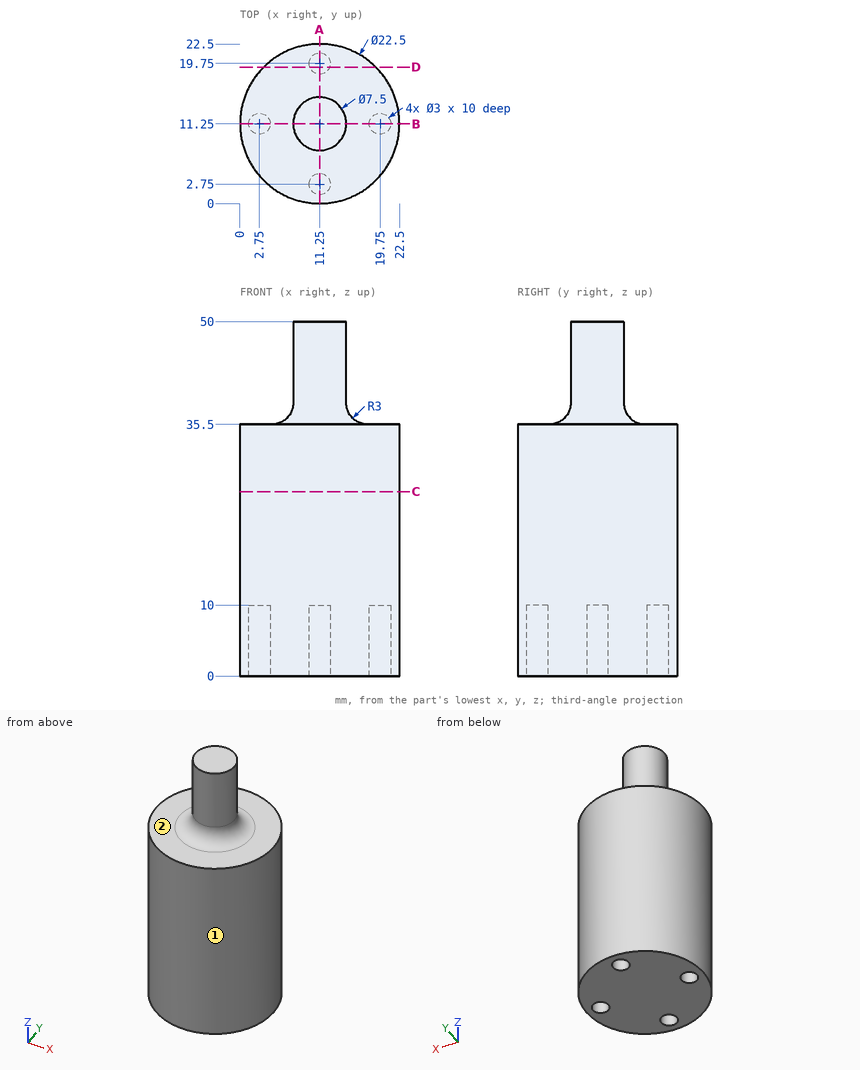
For this review, use the dimensioned drawing (mm, ordinates from the lowest corner) and the shaded views. A direction names the side the tool comes from. Round coordinates to 2 decimals unless told otherwise and drop trailing zeros. Order: outer loops, then holes, each group sorted by start corner. A loop starts at its lowest first (then second) coordinate and runs counter-clockwise, first axis right, second up. Notation, with made-up numbers: M 18.5,77 L 33.5,77 A26 cw 33.5,114 Z; hole C 40,42 d9. An arc over 180 degrees is marked long. Use a Markdown table: item, result. Add a question column.
Item 1: To check wall thickness, follow line 1 along Y through (x, z) = (11.25, 3); line 2 along Z through (x, y) = (10.25, 4.75); line 3 along Y through (x, z) = (19.75, 2.5). State the ranges of each line that lie inside material, in increasing order.
Item 2: Tool access review of the marked faces 1 and 2: name each direction out of +Z, -Z, +X, -X, +Y, -Y from which nothing blocks a thin tool from reaching the whole face with its end or side.
Item 3: Add section D-D, the plane y = 19.25. Give the boundary of the cut face in (x, z), then the cut area to 3 significant figures.
Item 4: Add section A-A, the plane x = 11.25. Give the boundary of the cut face in (y, z).
Item 5: Insertion check: pin 1 (6 mm diameter, centred on x = 2.5, y = 19, fed in from +Z); pin 2 (1.5 mm diameter, centred on y = 14, z = 38.5, fed in from +X); pin 3 (8 mm diameter, centred on y = 7, z = 43.5, fed in from -X). Each pin has a flat end and moves straight along its axis. Give the tip position at first contact, or say it passes through.
Item 6: Add section C-C, the plane z = 26. Give the boundary of the cut face in (x, y), then the cut area to 3 significant figures.
Geometry results:
| question | item | result |
|---|---|---|
| 1 | line 1 | y = 0 to 1.25, 4.25 to 18.25, 21.25 to 22.5 |
| 1 | line 2 | z = 0 to 35.51 |
| 1 | line 3 | y = 3.88 to 9.75, 12.75 to 18.62 |
| 2 | face 1 | +Z, -Z |
| 2 | face 2 | +Z |
| 3 | outline | M 3.34,0 L 9.84,0 L 9.84,10 L 12.66,10 L 12.66,0 L 19.16,0 L 19.16,35.5 L 3.34,35.5 Z |
| 3 | area | 533 mm² |
| 4 | outline | M 0,0 L 1.25,0 L 1.25,10 L 4.25,10 L 4.25,0 L 18.25,0 L 18.25,10 L 21.25,10 L 21.25,0 L 22.5,0 L 22.5,35.5 L 18,35.5 A3 cw 15,38.5 L 15,50 L 7.5,50 L 7.5,38.5 A3 cw 4.5,35.5 L 0,35.5 Z |
| 5 | pin 1 | stops at z = 35.5 |
| 5 | pin 2 | stops at x = 14.42 |
| 5 | pin 3 | stops at x = 7.51 |
| 6 | outline | C 11.25,11.25 d22.5 |
| 6 | area | 398 mm² |
